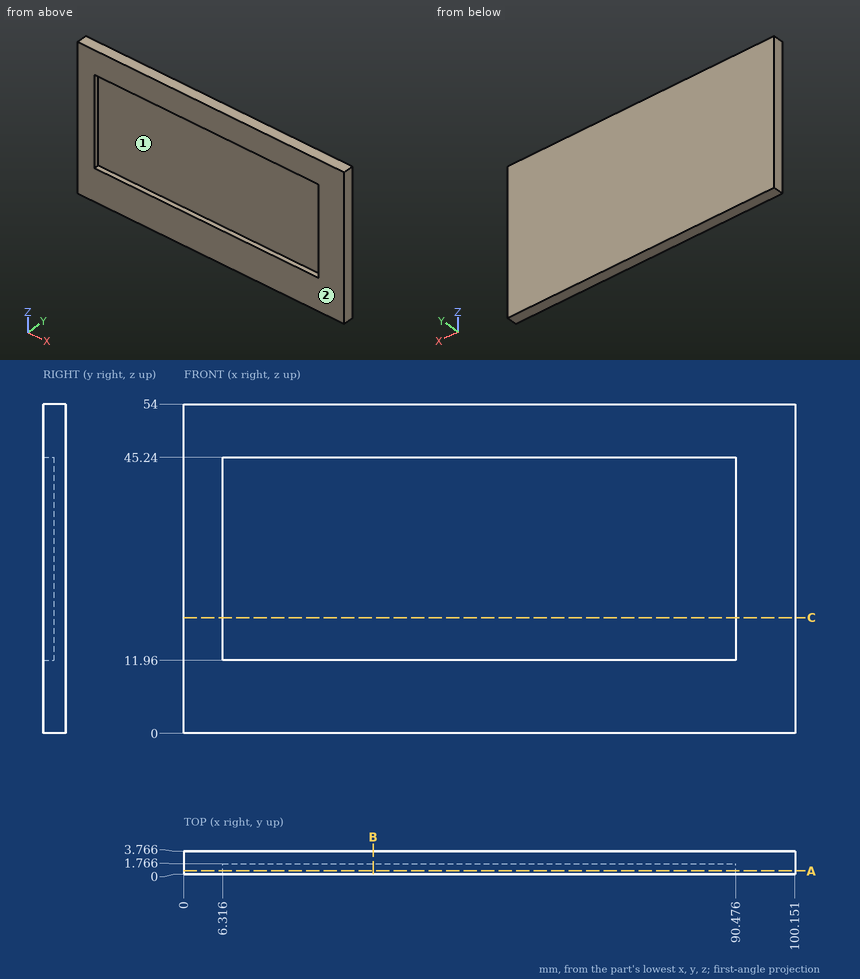
Verification items for this drawing (mm, ordinates from the low corner). A direction names the side the tool comes from. Round coordinates to 2 decimals unless told otherwise and drop trailing zeros. Order: outer loops, then holes, each group sorted by start corner. A loop starts at its lowest first (then second) coordinate and runs counter-clockwise, first axis right, second up. Notation, with made-up numbers: M 50.25,26 L 67.25,26 A37 ccw 67.25,65 Z; hole C -5,68 d10. An arc over 180 degrees is marked long. Answer in a Markdown table with one row per item. Add a question column.
Item 1: Material ranges on L1, parallel to Z at x = 51, y = 0.95; L2, parallel to Y at x = 70, z = 30 (1 decimal); L3, parallel to X at y = 0.3, z = 38 (1 decimal), recorded low to high. Write a range as [from, to].
Item 2: Sectioned sample at B-B, the plane x = 31. Enter the section's corners in (y, z) (1 decimal).
Item 3: Depth check by flat-ended pin: pin 1 Ø5 at (x, z) = (20.5, 33.5) entering from -Y. Enter the tip coordinate at first touch or a pass-through.
Item 4: Sectioned sample at A-A, the plane y = 0.6. Enter the section's corners in (x, z) (1 decimal).
Item 5: Set-up check for the marked faces 1 and 2: record each of +Z, -Z, +X, -X, +Y, -Y from which the full face is reachable in a straight line by a thin tool's end or side.
Item 6: Sectioned sample at C-C, the plane z = 19. Enter the section's corners in (x, y) (1 decimal).
Filled in:
| question | item | result |
|---|---|---|
| 1 | L1 | z = [0, 11.96], [45.24, 54] |
| 1 | L2 | y = [1.8, 3.8] |
| 1 | L3 | x = [0, 6.3], [90.5, 100.2] |
| 2 | outline | M 0,0 L 3.8,0 L 3.8,54 L 0,54 L 0,45.2 L 1.8,45.2 L 1.8,12 L 0,12 Z |
| 3 | pin 1 | stops at y = 1.77 |
| 4 | outline | M 0,0 L 100.2,0 L 100.2,54 L 0,54 Z; hole M 6.3,12 L 90.5,12 L 90.5,45.2 L 6.3,45.2 Z |
| 5 | face 1 | -Y |
| 5 | face 2 | +Z, -Z, +X, -X, -Y |
| 6 | outline | M 0,0 L 6.3,0 L 6.3,1.8 L 90.5,1.8 L 90.5,0 L 100.2,0 L 100.2,3.8 L 0,3.8 Z |
